```python
from build123d import *

# Parameters (mm, degrees)
BOSS_EXTRU_1_DEPTH         = 10
ESQUISSE2_W                = 10
ESQUISSE2_H                = 10
ENL_V_MAT_EXTRU_1_DEPTH    = 10
R_P_TITION_LIN_AIRE1_COUNT = 3
R_P_TITION_LIN_AIRE1_PITCH = 20


with BuildPart() as part:
    # Esquisse1 → Boss.-Extru.1 (new body)
    with BuildSketch(Plane(origin=(0, 0, 0), x_dir=(0, 0, -1), z_dir=(1, 0, 0))):
        Polygon((0, -300), (-20, -300), (-20, -73), (-130, -73), (-130, -300), (-150, -300), (-150, 0), (0, 0), align=None)
    extrude(amount=BOSS_EXTRU_1_DEPTH)

    # Esquisse2 → Enlèv. mat.-Extru.1 (cut)
    with BuildSketch(Plane(origin=(10, 0, 0), x_dir=(0, 0, -1), z_dir=(1, 0, 0))):
        with Locations((-5, -15)):
            Rectangle(ESQUISSE2_W, ESQUISSE2_H)
    enl_v_mat_extru_1 = extrude(amount=-ENL_V_MAT_EXTRU_1_DEPTH, mode=Mode.SUBTRACT)

    # Répétition linéaire1: Enlèv. mat.-Extru.1 ×3
    with Locations(*[(0, -i * R_P_TITION_LIN_AIRE1_PITCH, 0) for i in range(1, R_P_TITION_LIN_AIRE1_COUNT)]):
        add(enl_v_mat_extru_1, mode=Mode.SUBTRACT)


solid = part.part
```
For this review, take the finished solid that the model builds, in its own axes (mm). A direction names the side the tool comes from. Coordinates: 2 decimals unless noted, no trailing zeros. Write each loop counter-clockwise with the first axis right and the second up, starting at its lowest first coordinate (ties: lowest second). Pieces come first, ordered by that corner, then holes.
(1) Add section B-B on x = 7.75. Give the boundary of the cut face in (y, z).
(2) Add section C-C on z = 48.5. Give the boundary of the cut face in (x, y), then the cut area to 3 significant figures.
(3) Add section A-A on y = -136. Give the boundary of the cut face in (x, z), then the cut area to 3 significant figures.
(4) The part is to be moulded in two halves that separate along Y. For faces 4 (the face through (5, -300, 10)), 5 (the face through (5, -20, 5)), 6 (the face through (5, -15, 10)), 7 (the face through (5, -45, 0)), say which applies: +Y half, -Y half, draft (parallel to the pull), parting line (faces both ways), or undercut.
(5) Wall thickness on probe 1 along Y at (x, z) = (7.75, 7); probe 2 along Z at (x, y) = (4, -275.5); probe 3 along Z at (x, y) = (2.5, -34): over which ranges is each line inside the solid? List them lowest first.
(6) For pin 1 Ø4 at (x, y) = (1.5, -159) entering from -Z; pin 2 Ø1 at (x, y) = (6.5, -37) entering from -Z; pin 3 Ø1 at (x, z) = (8.5, 42.5) entering from -Y, all flat-tipped, find the tip position at first contact; note any pin that passes through.
(7) Tool access review of faces 1 (the face through (5, -188, 20)), 2 (the face through (5, -40, 5)), 3 (the face through (10, -48, 74)): name each direction out of +Z, -Z, +X, -X, +Y, -Y from which nothing blocks a thin tool from reaching the whole face with its end or side.
Answer sheet:
1. outline: (-300, 0) - (-60, 0) - (-60, 10) - (-50, 10) - (-50, 0) - (-40, 0) - (-40, 10) - (-30, 10) - (-30, 0) - (-20, 0) - (-20, 10) - (-10, 10) - (-10, 0) - (0, 0) - (0, 150) - (-300, 150) - (-300, 130) - (-73, 130) - (-73, 20) - (-300, 20) - close
2. outline: (0, -73) - (10, -73) - (10, 0) - (0, 0) - close
2. area: 730 mm2
3. outline: (0, 0) - (10, 0) - (10, 20) - (0, 20) - close; (0, 130) - (10, 130) - (10, 150) - (0, 150) - close
3. area: 400 mm2
4. face 4: -Y half
4. face 5: undercut
4. face 6: undercut
4. face 7: draft
5. probe 1: y = -300 to -60, -50 to -40, -30 to -20, -10 to 0
5. probe 2: z = 0 to 20, 130 to 150
5. probe 3: z = 10 to 150
6. pin 1: stops at z = 0
6. pin 2: stops at z = 10
6. pin 3: stops at y = -73
7. face 1: +X, -X, -Y
7. face 2: -Z, +X, -X
7. face 3: +Z, -Z, +X, +Y, -Y
